Solid Edge part; units mm, degrees
sketch "Sketch1" plane through (0, 0, 0) normal (0, 0, 1) x (1, 0, 0)
  circle A0 centre (0, 0) radius 12.7
  circle A1 centre (0, 9.5) radius 1.5
  circle A2 centre (-8.2272, -4.75) radius 1.5
  circle A3 centre (8.2272, -4.75) radius 1.5
extrude "Protrusion1" add sketch "Sketch1" along normal blind 4
sketch "Sketch2" plane through (0, 0, 4) normal (0, 0, 1) x (0, 1, 0)
  circle A0 centre (4, 6.9282) radius 2.425
  circle A1 centre (4, -6.9282) radius 2.425
  circle A2 centre (-8, 0) radius 2.425
extrude "ExtrudedProtrusion_3" add sketch "Sketch2" along normal blind 20
Input: part model. Units: mm. Frame: model coordinates. A direction names the side the tool comes from. Give positions to 0.01 mm unless a question says otherwise; leave off trailing zeros. Write each loop counter-clockwise with the first axis right and the second up, starting at its lowest first coordinate (ties: lowest second). Pieces come first, ordered by that corner, then holes. Notation, with made-up numbers: M 43.25,-22.5 L 52.25,-22.5 A24 ccw 52.25,16.5 Z; hole C 28.5,78 d3. An arc over 180 degrees is marked long. Use one line per item in the form item = value.
1. Mould query, pull axis X, two halves, no side actions, for faces 1 (the face through (0, 11, 2)), 2 (the face through (0, 0, 0)), 3 (the face through (0.107, -10.423, 13.86)). Classes: released by +X, released by -X, zero draft, split by the parting line, or undercut.
Outcome:
face_1 = undercut
face_2 = zero draft
face_3 = split by the parting line
2. Reachability of faces 4 (the face through (-9.726, -4.816, 1.972)), 5 (the face through (0, 0, 4)) from +Z, -Z, +X, -X, +Y, -Y: full face, straight path, thin tool, end or side. Return the list, or none.
Outcome:
face_4 = +Z, -Z
face_5 = +Z
3. Cut plane D-D on y = -8. Return loops of the section in (x, z) (3 decimals).
Outcome:
outline = M -9.864,0 L 9.864,0 L 9.864,4 L 2.425,4 L 2.425,24 L -2.425,24 L -2.425,4 L -9.864,4 Z
4. Ray query, L1, parallel to Z at x = 0.25, y = 3.75; L2, parallel to Y at x = 0, z = 1.6; L3, parallel to Y at x = 2, z = 17.5. Return the intervals inside material, ascending.
Outcome:
L1 = 0 to 4
L2 = -12.7 to 8, 11 to 12.7
L3 = -9.37 to -6.63
5. Cut plane B-B on y = 9.5. Return loops of the section in (x, z), and give its area (3 significant figures).
Outcome:
outline = M -8.43,0 L -1.5,0 L -1.5,4 L -8.43,4 Z; M 1.5,0 L 8.43,0 L 8.43,4 L 1.5,4 Z
area = 55.4 mm²
6. Cut plane A-A on x = 0. Return loops of the section in (y, z) (3 decimals).
Outcome:
outline = M -12.7,0 L 8,0 L 8,4 L -5.575,4 L -5.575,24 L -10.425,24 L -10.425,4 L -12.7,4 Z; M 11,0 L 12.7,0 L 12.7,4 L 11,4 Z
7. Cut plane C-C on z = 7.75. Return loops of the section in (x, y) (3 decimals), and give its area (3 significant figures).
Outcome:
outline = C -6.928,4 d4.85; C 0,-8 d4.85; C 6.928,4 d4.85
area = 55.4 mm²
8. First-contact query: P1, Ø5, axis at x = 0.5, y = -8.5, coming from the -Z side; P2, Ø3, axis at x = -5, z = 16, coming from the -Y side; P3, Ø2, axis at x = 5.5, z = 21, coming from the +Y side; P4, Ø3.5, axis at x = 0, y = 9.5, coming from the +Z side. Flat tips, straight axial feed; report the tip coordinate or a pass-through.
Outcome:
P1 = 0
P2 = 1.61
P3 = 6.39
P4 = 4
